Verification items for the finished model (mm, model axes). Coordinates: 2 decimals unless noted, no trailing zeros. Order: outer loops, then holes, each group sorted by start corner. A loop starts at its lowest first (then second) coordinate and runs counter-clockwise, first axis right, second up. Notation, with made-up numbers: M 9.25,53.5 L 28.25,53.5 A33 cw 28.25,87.5 Z; hole C -2.75,70.5 d1. An arc over 180 degrees is marked long. Use one line per item in the form item = value. Start each with the question number.
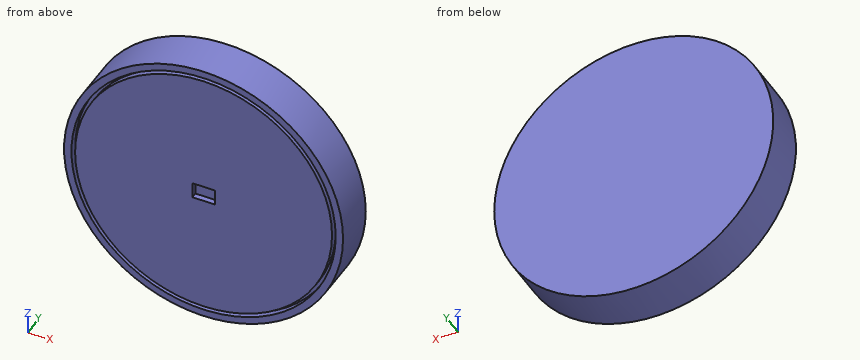
```python
from build123d import *

# Parameters (mm, degrees)
SKETCH1_R           = 60.325
BOSS_EXTRUDE1_DEPTH = 19.05
SKETCH2_R           = 57.15
SKETCH2_R_2         = 55.5625
CUT_EXTRUDE1_DEPTH  = 3.175
SKETCH3_W           = 9.697234664
SKETCH3_H           = 6.926230082
CUT_EXTRUDE2_DEPTH  = 2.54


with BuildPart() as part:
    # Sketch1 → Boss-Extrude1 (new body)
    with BuildSketch(Plane(origin=(0, 0, 0), x_dir=(1, 0, 0), z_dir=(0, 1, 0))):
        Circle(SKETCH1_R)
    extrude(amount=BOSS_EXTRUDE1_DEPTH)

    # Sketch2 → Cut-Extrude1 (cut)
    with BuildSketch(Plane.XZ):
        Circle(SKETCH2_R)
        Circle(SKETCH2_R_2, mode=Mode.SUBTRACT)
    extrude(amount=-CUT_EXTRUDE1_DEPTH, mode=Mode.SUBTRACT)

    # Sketch3 → Cut-Extrude2 (cut)
    with BuildSketch(Plane.XZ):
        Rectangle(SKETCH3_W, SKETCH3_H)
    extrude(amount=-CUT_EXTRUDE2_DEPTH, mode=Mode.SUBTRACT)


solid = part.part
```
1. Depth check by flat-ended pin: P1, Ø1.5, axis at y = 17, z = -36, coming from the -X side; P2, Ø1, axis at y = 5.5, z = -16.5, coming from the +X side; P3, Ø3, axis at y = 5.5, z = 40.5, coming from the -X side. Enter the tip coordinate at first touch or a pass-through.
2. Cross-section at D-D on x = -11. Enter the section's corners in (y, z) (3 decimals).
3. Cross-section at C-C on y = 13. Enter the section's corners in (x, z) (3 decimals), and give its area (3 significant figures).
4. Cross-section at B-B on x = -31.5. Enter the section's corners in (y, z) (3 decimals).
5. Material ranges on line 1 along X through (y, z) = (1.5, -0.5); line 2 along X through (y, z) = (2.25, 2) (1 decimal); line 3 along X through (y, z) = (1.25, -30), recorded low to high.
Final values:
q1.P1 = -48.95
q1.P2 = 58.16
q1.P3 = -46.02
q2.outline = M 0,-59.314 L 19.05,-59.314 L 19.05,59.314 L 0,59.314 L 0,56.081 L 3.175,56.081 L 3.175,54.463 L 0,54.463 L 0,-54.463 L 3.175,-54.463 L 3.175,-56.081 L 0,-56.081 Z
q3.outline = C 0,0 d120.65
q3.area = 11,400 mm2
q4.outline = M 0,-51.448 L 19.05,-51.448 L 19.05,51.448 L 0,51.448 L 0,47.685 L 3.175,47.685 L 3.175,45.771 L 0,45.771 L 0,-45.771 L 3.175,-45.771 L 3.175,-47.685 L 0,-47.685 Z
q5.line_1 = -60.32 to -57.15, -55.56 to -4.85, 4.85 to 55.56, 57.15 to 60.32
q5.line_2 = -60.3 to -57.1, -55.5 to -4.8, 4.8 to 55.5, 57.1 to 60.3
q5.line_3 = -52.34 to -48.64, -46.77 to 46.77, 48.64 to 52.34
